Can you work these out from the model? Positions are in its coordinate system, mm. A direction names the side the tool comes from. Give positions to 0.01 mm unless a question says otherwise; leave off trailing zeros. Order: outer loops, then holes, each group sorted by start corner. A loop starts at its lowest first (then second) coordinate and runs counter-clockwise, first axis right, second up. Notation, with made-up numbers: (73, 51) - (89, 51) arc R17 cw to (89, 77) - close; hole circle Ø8 at (66.25, 15.25). An arc over 180 degrees is marked (long way). Answer as CSV lines item,"result".
Autodesk Inventor part; units mm, degrees
ref_plane "YZ Plane" through (0, 0, 0) normal (1, 0, 0) x (0, 1, 0)
ref_plane "XZ Plane" through (0, 0, 0) normal (0, 1, 0) x (-1, 0, 0)
ref_plane "XY Plane" through (0, 0, 0) normal (0, 0, 1) x (1, 0, 0)
sketch "Sketch1" plane through (0, 0, 0) normal (0, 0, 1) x (1, 0, 0)
  circle A0 centre (0, 0) radius 3.675
  circle A1 centre (0, 0) radius 6.35
  line L0 (-10.287, 10.287) -> (10.287, 10.287)
  line L1 (10.287, 10.287) -> (10.287, -10.287)
  line L2 (-10.287, -10.287) -> (-10.287, 10.287)
  line L3 (10.287, 10.287) -> (0, 10.287) construction
  circle A2 centre (-6.9596, 6.9596) radius 1.3716
  line L4 (-6.9596, 6.9596) -> (-10.287, 10.287) construction
  circle A3 centre (6.9596, 6.9596) radius 1.3716
  line L5 (6.9596, 6.9596) -> (10.287, 10.287) construction
  line L6 (-6.9596, 6.9596) -> (6.9596, 6.9596) construction
  circle A4 centre (-6.9596, -6.9596) radius 1.3716
  circle A5 centre (6.9596, -6.9596) radius 1.3716
  line L7 (-6.9596, 6.9596) -> (-6.9596, -6.9596) construction
  line L8 (-10.287, -10.287) -> (-8.2403, -10.287)
  line L9 (10.287, -10.287) -> (8.2403, -10.287)
  line L10 (21.5842, 10.287) -> (21.5842, 0) construction
  line L11 (21.5842, 0) -> (21.5842, -10.287) construction
  arc A6 (-4.7625, -13.7648) -> (-8.2403, -10.287) centre (-8.2403, -13.7648) ccw
  arc A7 (8.2403, -10.287) -> (4.7625, -13.7648) centre (8.2403, -13.7648) ccw
  line L12 (-4.7625, -13.7648) -> (-4.7625, -17.8424)
  line L13 (4.7625, -13.7648) -> (4.7625, -17.8424)
  line L14 (-4.7625, -17.8424) -> (4.7625, -17.8424)
  line L15 (0, -17.1877) -> (-4.7625, -17.1877) construction
  line L16 (0, -17.1877) -> (4.7625, -17.1877) construction
  point P0 (0, 10.287)
  dimension "d7" = 7.35
  dimension "d8" = 12.7
  dimension "d11" = 10.287
  dimension "d14" = 20.574
  dimension "d15" = 2.7432
  dimension "d16" = 45
  dimension "d18" = 2.7432
  dimension "d19" = 45
  dimension "d20" = 13.9192
  dimension "d21" = 2.7432
  dimension "d22" = 2.7432
  dimension "d23" = 13.9192
  dimension "d25" = 20.574
  dimension "d27" = 20.574
  dimension "d28" = 10.287
  dimension "d34" = 9.525
  dimension "d44" = 4.7625
extrude "Extrusion1" add sketch "Sketch1" along normal blind 7.62 contours A1 | L0 L1 L9 A7 L13 L14 L12 A6 L8 L2
sketch "Sketch2" plane through (0, 0, 7.62) normal (0, 0, 1) x (1, 0, 0)
  circle A0 centre (0, 0) radius 3.675
  circle A1 centre (0, 0) radius 6.35
  dimension "d37" = 12.7
extrude "Extrusion2" add sketch "Sketch2" along normal blind 2.54
fillet "Fillet1" radius 1.905 1 edges at (10.287, 10.287, 3.81)
fillet "Fillet2" radius 1.905 1 edges at (-10.287, 10.287, 3.81)
fillet "Fillet3" radius 1.905 1 edges at (-10.287, -10.287, 3.81)
fillet "Fillet4" radius 1.905 1 edges at (10.287, -10.287, 3.81)
sketch "Sketch3" plane through (0, 0, 0) normal (0, 0, -1) x (-1, 0, 0)
  line L0 (-4.7625, -13.7648) -> (-4.7625, -17.8424)
  line L1 (-4.7625, -17.8424) -> (4.7625, -17.8424)
  line L2 (4.7625, -17.8424) -> (4.7625, -13.7648)
  line L3 (-10.287, 8.382) -> (-10.287, -8.382)
  circle A0 centre (0, 0) radius 3.675
  line L4 (-4.7625, -17.8424) -> (-0.9525, -17.8424) construction
  line L5 (4.7625, -16.7338) -> (0.9525, -16.7338) construction
  line L6 (-0.9525, -17.8424) -> (-0.9525, -3.5494)
  line L7 (0.9525, -17.8424) -> (0.9525, -3.5494)
  line L8 (-0.9525, -17.8424) -> (0.9525, -17.8424)
  arc A1 (-0.9525, -3.5494) -> (0.9525, -3.5494) centre (0, 0) ccw
  dimension "d45" = 3.81
  dimension "d46" = 3.81
extrude "Extrusion3" cut sketch "Sketch3" against normal blind 10.16 contours L6 A0 L7 L1
equation "\"d11\" = 0.5 * d9"
equation "\"d14\" = d9"
equation "\"d18\" = d15"
equation "\"d19\" = d16"
equation "\"d21\" = d15"
equation "\"d22\" = d15"
equation "\"d23\" = d20"
equation "\"d25\" = d14"
equation "\"d27\" = d25"
equation "\"d28\" = 0.5 * d14"
equation "\"d44\" = 0.5 * d34"
equation "\"d46\" = d45"
properties part number "widget"
1) I want a section at A-A on y = 0. Write out the boundary of the cut face in (x, z) (3 decimals).
Answer block:
outline,"(-10.287, 0) - (-3.675, 0) - (-3.675, 10.16) - (-6.35, 10.16) - (-6.35, 7.62) - (-10.287, 7.62) - close; (3.675, 0) - (10.287, 0) - (10.287, 7.62) - (6.35, 7.62) - (6.35, 10.16) - (3.675, 10.16) - close"
2) I want a section at C-C on z = 2.75. Count the separate pieces of the cut face and the enclosed holes in it, plus the area to 3 significant figures.
Answer block:
separate pieces,"1"
enclosed holes,"4"
area,"404 mm2"
3) I need wall thicknesses on line 1 along X through (y, z) = (-8.5, 4.75); line 2 along X through (y, z) = (0, 7.25) (3 decimals); line 3 along Z through (x, y) = (-4.25, -14). Which ranges of each line are inside material? Lowest first, please. Write a range as [from, to].
Answer block:
line 1,"[-10.28, -0.95], [0.95, 10.28]"
line 2,"[-10.287, -3.675], [3.675, 10.287]"
line 3,"[0, 7.62]"
4) I'm going to push flat-ended pins straight in: P1, Ø3.5, axis at y = -16, z = 5.5, coming from the +X side; P2, Ø1.5, axis at x = -6, z = 9, coming from the -Y side; P3, Ø1.5, axis at x = -4.5, y = -8, coming from the +Z side. Where does each tip first touch, or does it pass through?
Answer block:
P1,"x = 4.76"
P2,"y = -3.57"
P3,"z = 7.62"
5) If we mould it in two halves opening along Y, with no side actions, what happens to faces 1 (the cylindrical face through (-5.65, 6.55, 3.76)), 2 (the cylindrical face through (9.714, -9.744, 3.863)), 3 (the cylindrical face through (-0.266, 6.344, 8.872))? For each: +Y half, -Y half, draft (parallel to the pull), parting line (faces both ways), or undercut.
Answer block:
face 1,"undercut"
face 2,"-Y half"
face 3,"parting line"
6) Which directions (+Z, -Z, +X, -X, +Y, -Y) give clear straight access to the entire face, cutting with the end or side of a thin tool? Please do faces 4 (the flat face through (2, -7, 7.62)), 5 (the flat face through (-0.952, -11, 4)), 6 (the cylindrical face through (5.59, -7.02, 3.76)).
Answer block:
face 4,"+Z"
face 5,"+Z, -Z, -Y"
face 6,"+Z, -Z"
7) I want a section at D-D on x = -6. Write out the boundary of the cut face in (y, z).
Answer block:
outline,"(-11.1, 0) - (-7.94, 0) - (-7.94, 7.62) - (-11.1, 7.62) - close; (-5.98, 0) - (5.98, 0) - (5.98, 7.62) - (2.08, 7.62) - (2.08, 10.16) - (-2.08, 10.16) - (-2.08, 7.62) - (-5.98, 7.62) - close; (7.94, 0) - (10.29, 0) - (10.29, 7.62) - (7.94, 7.62) - close"
8) I want a section at B-B on x = -3. Write out the boundary of the cut face in (y, z), plus the area to 3 significant figures.
Answer block:
outline,"(-17.84, 0) - (-2.12, 0) - (-2.12, 10.16) - (-5.6, 10.16) - (-5.6, 7.62) - (-17.84, 7.62) - close; (2.12, 0) - (10.29, 0) - (10.29, 7.62) - (5.6, 7.62) - (5.6, 10.16) - (2.12, 10.16) - close"
area,"200 mm2"
